```python
from build123d import *

# Parameters (mm, degrees)
PAD_DEPTH      = 7
PAD_DEPTH_BACK = 7
SKETCH720_R    = 2.8
POCKET_DEPTH   = 100


with BuildPart() as part:
    # Sketch719 → Pad (new body, two sides)
    with BuildSketch(Plane.XZ) as pad_sk:
        with BuildLine():
            Line((0.9, 32.8), (9, 32.8))
            Line((9, 32.8), (9, 6))
            Line((9, 6), (21, 6))
            Line((21, 6), (21, 0))
            Line((21, 0), (0, 0))
            Line((0, 0), (0, 16))
            ThreePointArc((0, 16), (3.974276, 19.547087), (0.9, 23.897435))
            Line((0.9, 32.8), (0.9, 23.897435))
        make_face()
    pad = extrude(amount=PAD_DEPTH) + extrude(pad_sk.sketch, amount=-PAD_DEPTH_BACK)

    # Mirrored: Pad across Sketch719 V_Axis
    add(pad.mirror(Plane(origin=(0, 0, 0), x_dir=(0, -1, 0), z_dir=(1, 0, 0))))

    # Sketch720 (on Face4 of Mirrored) → Pocket (cut)
    with BuildSketch(Plane(origin=(0, 0, 6), x_dir=(-1, 0, 0), z_dir=(0, 0, 1))):
        with Locations((16, 0)):
            Circle(SKETCH720_R)
        with Locations((-16, 0)):
            Circle(SKETCH720_R)
    extrude(amount=-POCKET_DEPTH, mode=Mode.SUBTRACT)


solid = part.part
```
Part model, mm, in its own coordinate system. A direction names the side the tool comes from. Round coordinates to 2 decimals unless told otherwise and drop trailing zeros. Write each loop counter-clockwise with the first axis right and the second up, starting at its lowest first coordinate (ties: lowest second). Pieces come first, ordered by that corner, then holes. Notation, with made-up numbers: M 7,46 L 23,46 A17 ccw 23,73 Z; hole C 13,13.5 d2. An arc over 180 degrees is marked long. Answer as CSV lines item,"result". Start each with the question number.
1) Band-saw the part on C-C (y = 0). List the corners of the cut face in (x, z), then the cut area to 3 significant figures.
2) Which spindle directions (+Z, -Z, +X, -X, +Y, -Y) get a long thin tool onto all of the face, cutting with end or side? Do faces 1 (the face through (-9, 0, 20)), 2 (the face through (12, 0, 6)), 3 (the face through (-5, 0, 32.8)). Say none if no direction does.
3) Drop flat-ended pins along their axis: pin 1 (1.5 mm diameter, centred on y = -2.5, z = 9, fed in from -X); pin 2 (3.5 mm diameter, centred on x = 15, y = -1, fed in from +Z); pin 3 (4 mm diameter, centred on y = 3, z = 13.5, fed in from +X). Give the stop position or say it passes through.
4) Mould opens along X. For faces 4 (the face through (21, 0, 3)), 5 (the face through (0, 0, 0)), 6 (the face through (0.9, 0, 28)), 7 (the face through (-0.9, 0, 28)) say: +X half, -X half, draft (parallel to the pull), parting line (faces both ways), or undercut.
5) Band-saw the part on B-B (x = -16). List the corners of the cut face in (y, z).
6) Band-saw the part on D-D (y = -4). List the corners of the cut face in (x, z).
7) Band-saw the part on A-A (z = 27.5). List the corners of the cut face in (x, y).
8) Drill centre lines: L1, parallel to X at y = 0, z = 2.35; L2, parallel to Y at x = 16, z = 4.45; L3, parallel to X at y = -3, z = 26. Where is each one in solid material? Low to high.
Worked out:
1,outline,"M -21,0 L -18.8,0 L -18.8,6 L -21,6 Z; M -13.2,0 L 13.2,0 L 13.2,6 L 9,6 L 9,32.8 L 0.9,32.8 L 0.9,23.9 A4 cw long -0.9,23.9 L -0.9,32.8 L -9,32.8 L -9,6 L -13.2,6 Z; M 18.8,0 L 21,0 L 21,6 L 18.8,6 Z"
1,area,"601 mm²"
2,face 1,"+Z, -X, +Y, -Y"
2,face 2,"+Z, +X, +Y, -Y"
2,face 3,"+Z, +X, -X, +Y, -Y"
3,pin 1,"x = -9"
3,pin 2,"z = 6"
3,pin 3,"x = 9"
4,face 4,"+X half"
4,face 5,"draft"
4,face 6,"undercut"
4,face 7,"undercut"
5,outline,"M -7,0 L -2.8,0 L -2.8,6 L -7,6 Z; M 2.8,0 L 7,0 L 7,6 L 2.8,6 Z"
6,outline,"M -21,0 L 21,0 L 21,6 L 9,6 L 9,32.8 L 0.9,32.8 L 0.9,23.9 A4 cw long -0.9,23.9 L -0.9,32.8 L -9,32.8 L -9,6 L -21,6 Z"
7,outline,"M -9,-7 L -0.9,-7 L -0.9,7 L -9,7 Z; M 0.9,-7 L 9,-7 L 9,7 L 0.9,7 Z"
8,L1,"-21 to -18.8, -13.2 to 13.2, 18.8 to 21"
8,L2,"-7 to -2.8, 2.8 to 7"
8,L3,"-9 to -0.9, 0.9 to 9"
